Design review of the part built by this model. Coordinates are the model's own, in mm. A direction names the side the tool comes from. Coordinates: 2 decimals unless noted, no trailing zeros. Write each loop counter-clockwise with the first axis right and the second up, starting at its lowest first coordinate (ties: lowest second). Pieces come first, ordered by that corner, then holes.
Q1. Take a section at B-B, the plane x = 16.5. Write out the cut boundary in (y, z).
Q2. Take a section at A-A, the plane z = -8.5. Write out the cut boundary in (x, y).
Q3. For pin 1 Ø12 at (x, z) = (2, 9) entering from -Y; pin 2 Ø1.5 at (x, z) = (-11, -16) entering from +Y; pin 3 Ø4 at (y, z) = (5, -14) entering from +X; pin 4 Ø4 at (x, z) = (-14.72, -8.5) entering from -Y, all flat-tipped, find the tip position at first contact; note any pin that passes through.
Q4. For L1, parallel to Z at x = -13.5, y = 7.75; L2, parallel to X at y = 5.5, z = 8.5; L3, parallel to Y at x = 5, z = -19, list the stretches that pass through material, from the lowest coordinate up.
Q5. Take a section at C-C, the plane z = -17. Write out the cut boundary in (x, y), plus the area to 3 significant figures.
Q6. Take a section at D-D, the plane y = 6.75. Write out the cut boundary in (x, z).
Q7. For faces 5 (the cylindrical face through (-17.163, 4.93, 7.958)), 6 (the cylindrical face through (3.755, 17.395, 11.923)), list the 3-axis set-ups (+Z, -Z, +X, -X, +Y, -Y) from which the entire face can be reached by the end or side of a thin tool; tool diameter is ignored.
Q8. The part is to be moulded in two halves that separate along Z. For faces 1 (the cylindrical face through (6.31, 4.93, 20.03)), 2 (the cylindrical face through (0.1, 4.9, -19.5)), 3 (the flat face through (-9, 10, 9)), 4 (the cylindrical face through (-4.88, 12.66, -1.08)), say which applies: released by +Z, released by -Z, zero draft, split by the parting line, or undercut.
from build123d import *

# Parameters (mm, degrees)
SKETCH1_R           = 21
SKETCH1_R_2         = 2.5
BOSS_EXTRUDE1_DEPTH = 10
SKETCH2_R           = 12.5
BOSS_EXTRUDE2_DEPTH = 15
SKETCH3_R           = 5
CUT_EXTRUDE1_DEPTH  = 39.820097888
CHAMFER1_SIZE       = 1


with BuildPart() as part:
    # Sketch1 → Boss-Extrude1 (new body)
    with BuildSketch(Plane(origin=(0, 0, 0), x_dir=(1, 0, 0), z_dir=(0, 1, 0))):
        with Locations(Location((0, 0, 0), (0, 0, 270))):
            Circle(SKETCH1_R)
        with Locations(Location((0, 17, 0), (0, 0, 270))):
            Circle(SKETCH1_R_2, mode=Mode.SUBTRACT)
        with Locations(Location((14.722431864, 8.5, 0), (0, 0, 270))):
            Circle(SKETCH1_R_2, mode=Mode.SUBTRACT)
        with Locations(Location((14.722431864, -8.5, 0), (0, 0, 270))):
            Circle(SKETCH1_R_2, mode=Mode.SUBTRACT)
        with Locations(Location((0, -17, 0), (0, 0, 270))):
            Circle(SKETCH1_R_2, mode=Mode.SUBTRACT)
        with Locations(Location((-14.722431864, -8.5, 0), (0, 0, 270))):
            Circle(SKETCH1_R_2, mode=Mode.SUBTRACT)
        with Locations(Location((-14.722431864, 8.5, 0), (0, 0, 270))):
            Circle(SKETCH1_R_2, mode=Mode.SUBTRACT)
    extrude(amount=BOSS_EXTRUDE1_DEPTH)

    # Sketch2 → Boss-Extrude2 (add)
    with BuildSketch(Plane(origin=(0, 10, 0), x_dir=(1, 0, 0), z_dir=(0, 1, 0))):
        with Locations(Location((0, 0, 0), (0, 0, 270))):
            Circle(SKETCH2_R)
    extrude(amount=BOSS_EXTRUDE2_DEPTH)

    # Sketch3 → Cut-Extrude1 (cut, through all)
    with BuildSketch(Plane(origin=(0, 25, 0), x_dir=(1, 0, 0), z_dir=(0, 1, 0))):
        with Locations(Location((0, 0, 0), (0, 0, 270))):
            Circle(SKETCH3_R)
    extrude(amount=-CUT_EXTRUDE1_DEPTH, mode=Mode.SUBTRACT)

    # Chamfer1
    chamfer1_edges = [part.edges().sort_by_distance(p)[0] for p in [
        (0, 0, -5),
        (0, 25, -5),
    ]]
    chamfer(chamfer1_edges, length=CHAMFER1_SIZE)


solid = part.part
Responses:
1. outline: (0, -12.99) - (10, -12.99) - (10, -10.26) - (0, -10.26) - close; (0, -6.74) - (10, -6.74) - (10, 6.74) - (0, 6.74) - close; (0, 10.26) - (10, 10.26) - (10, 12.99) - (0, 12.99) - close
2. outline: (-19.2, 0) - (-17.22, 0) - (-17.22, 10) - (-19.2, 10) - close; (-12.22, 0) - (12.22, 0) - (12.22, 10) - (9.17, 10) - (9.17, 25) - (-9.17, 25) - (-9.17, 10) - (-12.22, 10) - close; (17.22, 0) - (19.2, 0) - (19.2, 10) - (17.22, 10) - close
3. pin 1: stops at y = 0
3. pin 2: stops at y = 10
3. pin 3: stops at x = 17.23
3. pin 4: passes through
4. L1: z = -16.09 to -10.68, -6.32 to 6.32, 10.68 to 16.09
4. L2: x = -19.2 to -17.22, -12.22 to 12.22, 17.22 to 19.2
4. L3: y = 0 to 10
5. outline: (-12.33, 0) - (-2.5, 0) - (-2.5, 10) - (-12.33, 10) - close; (2.5, 0) - (12.33, 0) - (12.33, 10) - (2.5, 10) - close
5. area: 197 mm2
6. outline: circle Ø42 at (0, 0); hole circle Ø5 at (-14.72, -8.5); hole circle Ø5 at (-14.72, 8.5); hole circle Ø10 at (0, 0); hole circle Ø5 at (0, -17); hole circle Ø5 at (0, 17); hole circle Ø5 at (14.72, -8.5); hole circle Ø5 at (14.72, 8.5)
7. face 5: +Y, -Y
7. face 6: +Y
8. face 1: split by the parting line
8. face 2: undercut
8. face 3: zero draft
8. face 4: undercut
